CAD build for the part. Positions are in the model's coordinates, mm. Round coordinates to 2 decimals unless told otherwise and drop trailing zeros. Write each loop counter-clockwise with the first axis right and the second up, starting at its lowest first coordinate (ties: lowest second). Pieces come first, ordered by that corner, then holes. Notation, with made-up numbers: (-19, 39.25) - (39, 39.25) arc R14 cw to (39, 64.25) - close; hole circle Ø8 at (-2, -10.75). An arc over 180 degrees is marked (long way). Put each result on its own line as item: value. Start each with the question number.
Item 1: Cut at C-C (z = 2.4). Give the cut face in (x, y) (3 decimals).
Item 2: Drill centre lines: line 1 (Y direction, x = -12.15, z = 2.1) (3 decimals); line 2 (Y direction, x = -5.5, z = 0.6); line 3 (X direction, y = 32.5, z = 3.7). Where is each one in solid material? Low to high. Write a range as from..to.
Item 3: Mould opens along X. For faces 1 (the cylindrical face through (-6.076, 34.294, 2.528)), 2 (the flat face through (-4, 9.751, 2)), 3 (the cylindrical face through (-12.38, 33.26, 2.47)) say: released by +X, released by -X, zero draft, split by the parting line, or undercut.
Item 4: Cut at A-A (x = -12.15). Give the cut face in (y, z) (3 decimals), and give its area (3 significant figures).
Item 5: Cut at B-B (y = 6). Give the cut face in (x, z).
Item 6: Pin check, flat tips, straight feed: pin 1 Ø1.2 at (x, z) = (-4, 3) entering from -Y; pin 2 Ø4 at (x, y) = (-4, 12.49) entering from +Z; pin 3 Ø2 at (y, z) = (4.5, 2) entering from +X. Stop position of each tip, or through.
Item 7: Cut at D-D (x = -4). Give the cut face in (y, z), and give its area (3 significant figures).
```python
from build123d import *

# Parameters (mm, degrees)
SKIZZE1_R                       = 1.8
AUFSATZ_LINEAR_AUSTRAGEN1_DEPTH = 5
VERRUNDUNG1_R                   = 2
FASE1_SIZE                      = 0.5


with BuildPart() as part:
    # Skizze1 → Aufsatz-Linear austragen1 (new body)
    with BuildSketch(Plane.XY):
        Polygon((-0.2, 9.751346921), (-0.2, 28.627239348), (-6.022760652, 34.45), (-16.1, 34.45), (-16.1, 0.2), (-8.2, 0.2), (-8.2, 9.751346921), align=None)
        with Locations((-12.15, 31.475)):
            Circle(SKIZZE1_R, mode=Mode.SUBTRACT)
        with Locations((-4, 12.49111782)):
            Circle(SKIZZE1_R, mode=Mode.SUBTRACT)
    extrude(amount=AUFSATZ_LINEAR_AUSTRAGEN1_DEPTH)

    # Verrundung1
    verrundung1_edges = [part.edges().sort_by_distance(p)[0] for p in [
        (-8.2, 9.751346921, 2.5),
        (-8.2, 0.2, 2.5),
        (-16.1, 0.2, 2.5),
        (-16.1, 34.45, 2.5),
        (-6.022760652, 34.45, 2.5),
        (-0.2, 28.627239348, 2.5),
        (-0.2, 9.751346921, 2.5),
    ]]
    fillet(verrundung1_edges, radius=VERRUNDUNG1_R)

    # Fase1
    # the kernel refuses this chamfer: 0.5 mm, written as the material it takes off along each edge
    with BuildSketch(Plane(origin=(-12.15, 31.475, 0), x_dir=(1, 0, 0), z_dir=(0, -1, 0))) as fase1_piece_1:
        Polygon((1.8 + FASE1_SIZE, 0), (1.8, FASE1_SIZE), (1.8, 0), align=None)
    revolve(axis=Axis((-12.15, 31.475, 0), (0, 0, 1)), mode=Mode.SUBTRACT)
    with BuildSketch(Plane(origin=(-12.15, 31.475, 5), x_dir=(1, 0, 0), z_dir=(0, -1, 0))) as fase1_piece_2:
        Polygon((1.8 + FASE1_SIZE, 0), (1.8, -FASE1_SIZE), (1.8, 0), align=None)
    revolve(axis=Axis((-12.15, 31.475, 5), (0, 0, 1)), mode=Mode.SUBTRACT)
    with BuildSketch(Plane(origin=(-4, 12.49111782, 0), x_dir=(1, 0, 0), z_dir=(0, -1, 0))) as fase1_piece_3:
        Polygon((1.8 + FASE1_SIZE, 0), (1.8, FASE1_SIZE), (1.8, 0), align=None)
    revolve(axis=Axis((-4, 12.49111782, 0), (0, 0, 1)), mode=Mode.SUBTRACT)
    with BuildSketch(Plane(origin=(-4, 12.49111782, 5), x_dir=(1, 0, 0), z_dir=(0, -1, 0))) as fase1_piece_4:
        Polygon((1.8 + FASE1_SIZE, 0), (1.8, -FASE1_SIZE), (1.8, 0), align=None)
    revolve(axis=Axis((-4, 12.49111782, 5), (0, 0, 1)), mode=Mode.SUBTRACT)
    with BuildSketch(Plane(origin=(-0.2, 11.751346921, 0), x_dir=(0.027495876610586382, 0, 0.9996219169112968), z_dir=(0, 1, 0))) as fase1_piece_5:
        Polygon((FASE1_SIZE * 0.999621916911, -FASE1_SIZE * 0.0274958766106), (-FASE1_SIZE * 0.0274958766106, -FASE1_SIZE * 0.999621916911), (0, 0), align=None)
    extrude(amount=16.047465302, mode=Mode.SUBTRACT)
    with BuildSketch(Plane(origin=(-0.2, 11.751346921, 5), x_dir=(0.027495876610586403, 0, -0.9996219169112968), z_dir=(0, 1, 0))) as fase1_piece_6:
        Polygon((FASE1_SIZE * 0.999621916911, FASE1_SIZE * 0.0274958766106), (-FASE1_SIZE * 0.0274958766106, FASE1_SIZE * 0.999621916911), (0, 0), align=None)
    extrude(amount=16.047465302, mode=Mode.SUBTRACT)
    with BuildSketch(Plane(origin=(-6.2, 9.751346921, 0), x_dir=(0, 0.9996219169112968, -0.02749587661058639), z_dir=(1, 0, 0))) as fase1_piece_7:
        Polygon((FASE1_SIZE * 0.999621916911, FASE1_SIZE * 0.0274958766106), (-FASE1_SIZE * 0.0274958766106, FASE1_SIZE * 0.999621916911), (0, 0), align=None)
    extrude(amount=4, mode=Mode.SUBTRACT)
    with BuildSketch(Plane(origin=(-8.2, 2.2, 0), x_dir=(-0.9996219169112968, 0, -0.02749587661058639), z_dir=(0, 1, 0))) as fase1_piece_8:
        Polygon((FASE1_SIZE * 0.999621916911, FASE1_SIZE * 0.0274958766106), (-FASE1_SIZE * 0.0274958766106, FASE1_SIZE * 0.999621916911), (0, 0), align=None)
    extrude(amount=5.551346921, mode=Mode.SUBTRACT)
    with BuildSketch(Plane(origin=(-14.1, 0.2, 0), x_dir=(0, 0.9996219169112968, -0.027495876610586372), z_dir=(1, 0, 0))) as fase1_piece_9:
        Polygon((FASE1_SIZE * 0.999621916911, FASE1_SIZE * 0.0274958766106), (-FASE1_SIZE * 0.0274958766106, FASE1_SIZE * 0.999621916911), (0, 0), align=None)
    extrude(amount=3.9, mode=Mode.SUBTRACT)
    with BuildSketch(Plane(origin=(-16.1, 32.45, 0), x_dir=(0.9996219169112968, 0, -0.02749587661058639), z_dir=(0, -1, 0))) as fase1_piece_10:
        Polygon((FASE1_SIZE * 0.999621916911, FASE1_SIZE * 0.0274958766106), (-FASE1_SIZE * 0.0274958766106, FASE1_SIZE * 0.999621916911), (0, 0), align=None)
    extrude(amount=30.25, mode=Mode.SUBTRACT)
    with BuildSketch(Plane(origin=(-6.851187777, 34.45, 0), x_dir=(0, -0.9996219169112968, -0.027495876610586483), z_dir=(-1, 0, 0))) as fase1_piece_11:
        Polygon((FASE1_SIZE * 0.999621916911, FASE1_SIZE * 0.0274958766106), (-FASE1_SIZE * 0.0274958766106, FASE1_SIZE * 0.999621916911), (0, 0), align=None)
    extrude(amount=7.248812223, mode=Mode.SUBTRACT)
    with BuildSketch(Plane(origin=(-0.785786438, 29.213025785, 0), x_dir=(-0.7068394360706736, -0.7068394360706733, -0.027495876610586348), z_dir=(-0.7071067811865475, 0.7071067811865477, 0))) as fase1_piece_12:
        Polygon((FASE1_SIZE * 0.999621916911, FASE1_SIZE * 0.0274958766106), (-FASE1_SIZE * 0.0274958766106, FASE1_SIZE * 0.999621916911), (0, 0), align=None)
    extrude(amount=6.577772835, mode=Mode.SUBTRACT)
    with BuildSketch(Plane(origin=(-2.2, 27.798812223, 0), x_dir=(1, 0, 0), z_dir=(0, -1, 0))) as fase1_piece_13:
        Polygon((2 - FASE1_SIZE, 0), (2, FASE1_SIZE), (2, 0), align=None)
    revolve(axis=Axis((-2.2, 27.798812223, 0), (0, 0, 1)), revolution_arc=45, mode=Mode.SUBTRACT)
    with BuildSketch(Plane(origin=(-6.851187777, 32.45, 0), x_dir=(0.7071067811865487, 0.7071067811865465, 0), z_dir=(0.7071067811865465, -0.7071067811865487, 0))) as fase1_piece_14:
        Polygon((2 - FASE1_SIZE, 0), (2, FASE1_SIZE), (2, 0), align=None)
    revolve(axis=Axis((-6.851187777, 32.45, 0), (0, 0, 1)), revolution_arc=45, mode=Mode.SUBTRACT)
    with BuildSketch(Plane(origin=(-14.1, 32.45, 0), x_dir=(0, 1, 0), z_dir=(1, 0, 0))) as fase1_piece_15:
        Polygon((2 - FASE1_SIZE, 0), (2, FASE1_SIZE), (2, 0), align=None)
    revolve(axis=Axis((-14.1, 32.45, 0), (0, 0, 1)), revolution_arc=90, mode=Mode.SUBTRACT)
    with BuildSketch(Plane(origin=(-14.1, 2.2, 0), x_dir=(-1, 0, 0), z_dir=(0, 1, 0))) as fase1_piece_16:
        Polygon((2 - FASE1_SIZE, 0), (2, FASE1_SIZE), (2, 0), align=None)
    revolve(axis=Axis((-14.1, 2.2, 0), (0, 0, 1)), revolution_arc=90, mode=Mode.SUBTRACT)
    with BuildSketch(Plane(origin=(-10.2, 2.2, 0), x_dir=(0, -1, 0), z_dir=(-1, 0, 0))) as fase1_piece_17:
        Polygon((2 - FASE1_SIZE, 0), (2, FASE1_SIZE), (2, 0), align=None)
    revolve(axis=Axis((-10.2, 2.2, 0), (0, 0, 1)), revolution_arc=90, mode=Mode.SUBTRACT)
    with BuildSketch(Plane(origin=(-2.2, 11.751346921, 0), x_dir=(1, 0, 0), z_dir=(0, 1, 0))) as fase1_piece_18:
        Polygon((2 - FASE1_SIZE, 0), (2, -FASE1_SIZE), (2, 0), align=None)
    revolve(axis=Axis((-2.2, 11.751346921, 0), (0, 0, -1)), revolution_arc=90, mode=Mode.SUBTRACT)
    with BuildSketch(Plane(origin=(-6.2, 9.751346921, 5), x_dir=(0, 0.9996219169112968, 0.027495876610585647), z_dir=(1, 0, 0))) as fase1_piece_19:
        Polygon((FASE1_SIZE * 0.999621916911, -FASE1_SIZE * 0.0274958766106), (-FASE1_SIZE * 0.0274958766106, -FASE1_SIZE * 0.999621916911), (0, 0), align=None)
    extrude(amount=4, mode=Mode.SUBTRACT)
    with BuildSketch(Plane(origin=(-0.785786438, 29.213025785, 5), x_dir=(-0.7068394360706736, -0.7068394360706733, 0.027495876610585605), z_dir=(-0.7071067811865475, 0.7071067811865477, 0))) as fase1_piece_20:
        Polygon((FASE1_SIZE * 0.999621916911, -FASE1_SIZE * 0.0274958766106), (-FASE1_SIZE * 0.0274958766106, -FASE1_SIZE * 0.999621916911), (0, 0), align=None)
    extrude(amount=6.577772835, mode=Mode.SUBTRACT)
    with BuildSketch(Plane(origin=(-6.851187777, 34.45, 5), x_dir=(0, -0.9996219169112968, 0.02749587661058574), z_dir=(-1, 0, 0))) as fase1_piece_21:
        Polygon((FASE1_SIZE * 0.999621916911, -FASE1_SIZE * 0.0274958766106), (-FASE1_SIZE * 0.0274958766106, -FASE1_SIZE * 0.999621916911), (0, 0), align=None)
    extrude(amount=7.248812223, mode=Mode.SUBTRACT)
    with BuildSketch(Plane(origin=(-16.1, 32.45, 5), x_dir=(0.9996219169112968, 0, 0.027495876610585647), z_dir=(0, -1, 0))) as fase1_piece_22:
        Polygon((FASE1_SIZE * 0.999621916911, -FASE1_SIZE * 0.0274958766106), (-FASE1_SIZE * 0.0274958766106, -FASE1_SIZE * 0.999621916911), (0, 0), align=None)
    extrude(amount=30.25, mode=Mode.SUBTRACT)
    with BuildSketch(Plane(origin=(-14.1, 0.2, 5), x_dir=(0, 0.9996219169112968, 0.02749587661058563), z_dir=(1, 0, 0))) as fase1_piece_23:
        Polygon((FASE1_SIZE * 0.999621916911, -FASE1_SIZE * 0.0274958766106), (-FASE1_SIZE * 0.0274958766106, -FASE1_SIZE * 0.999621916911), (0, 0), align=None)
    extrude(amount=3.9, mode=Mode.SUBTRACT)
    with BuildSketch(Plane(origin=(-8.2, 2.2, 5), x_dir=(-0.9996219169112968, 0, 0.027495876610585647), z_dir=(0, 1, 0))) as fase1_piece_24:
        Polygon((FASE1_SIZE * 0.999621916911, -FASE1_SIZE * 0.0274958766106), (-FASE1_SIZE * 0.0274958766106, -FASE1_SIZE * 0.999621916911), (0, 0), align=None)
    extrude(amount=5.551346921, mode=Mode.SUBTRACT)
    with BuildSketch(Plane(origin=(-2.2, 27.798812223, 5), x_dir=(1, 0, 0), z_dir=(0, -1, 0))) as fase1_piece_25:
        Polygon((2, -FASE1_SIZE), (2 - FASE1_SIZE, 0), (2, 0), align=None)
    revolve(axis=Axis((-2.2, 27.798812223, 5), (0, 0, 1)), revolution_arc=45, mode=Mode.SUBTRACT)
    with BuildSketch(Plane(origin=(-6.851187777, 32.45, 5), x_dir=(0.7071067811865487, 0.7071067811865465, 0), z_dir=(0.7071067811865465, -0.7071067811865487, 0))) as fase1_piece_26:
        Polygon((2 - FASE1_SIZE, 0), (2, -FASE1_SIZE), (2, 0), align=None)
    revolve(axis=Axis((-6.851187777, 32.45, 5), (0, 0, 1)), revolution_arc=45, mode=Mode.SUBTRACT)
    with BuildSketch(Plane(origin=(-14.1, 32.45, 5), x_dir=(0, 1, 0), z_dir=(1, 0, 0))) as fase1_piece_27:
        Polygon((2 - FASE1_SIZE, 0), (2, -FASE1_SIZE), (2, 0), align=None)
    revolve(axis=Axis((-14.1, 32.45, 5), (0, 0, 1)), revolution_arc=90, mode=Mode.SUBTRACT)
    with BuildSketch(Plane(origin=(-14.1, 2.2, 5), x_dir=(-1, 0, 0), z_dir=(0, 1, 0))) as fase1_piece_28:
        Polygon((2 - FASE1_SIZE, 0), (2, -FASE1_SIZE), (2, 0), align=None)
    revolve(axis=Axis((-14.1, 2.2, 5), (0, 0, 1)), revolution_arc=90, mode=Mode.SUBTRACT)
    with BuildSketch(Plane(origin=(-10.2, 2.2, 5), x_dir=(0, -1, 0), z_dir=(-1, 0, 0))) as fase1_piece_29:
        Polygon((2 - FASE1_SIZE, 0), (2, -FASE1_SIZE), (2, 0), align=None)
    revolve(axis=Axis((-10.2, 2.2, 5), (0, 0, 1)), revolution_arc=90, mode=Mode.SUBTRACT)
    with BuildSketch(Plane(origin=(-2.2, 11.751346921, 5), x_dir=(1, 0, 0), z_dir=(0, 1, 0))) as fase1_piece_30:
        Polygon((2, FASE1_SIZE), (2 - FASE1_SIZE, 0), (2, 0), align=None)
    revolve(axis=Axis((-2.2, 11.751346921, 5), (0, 0, -1)), revolution_arc=90, mode=Mode.SUBTRACT)
    with BuildSketch(Plane(origin=(-6.2, 7.751346921, 0), x_dir=(-1, 0, 0), z_dir=(0, -1, 0))) as fase1_piece_31:
        Polygon((2 + FASE1_SIZE, 0), (2, -FASE1_SIZE), (2, 0), align=None)
    revolve(axis=Axis((-6.2, 7.751346921, 0), (0, 0, -1)), revolution_arc=90, mode=Mode.SUBTRACT)
    with BuildSketch(Plane(origin=(-6.2, 7.751346921, 5), x_dir=(-1, 0, 0), z_dir=(0, -1, 0))) as fase1_piece_32:
        Polygon((2 + FASE1_SIZE, 0), (2, FASE1_SIZE), (2, 0), align=None)
    revolve(axis=Axis((-6.2, 7.751346921, 5), (0, 0, -1)), revolution_arc=90, mode=Mode.SUBTRACT)


solid = part.part
```
Output values:
1. outline: (-16.1, 2.2) arc R2 ccw to (-14.1, 0.2) - (-10.2, 0.2) arc R2 ccw to (-8.2, 2.2) - (-8.2, 7.751) arc R2 cw to (-6.2, 9.751) - (-2.2, 9.751) arc R2 ccw to (-0.2, 11.751) - (-0.2, 27.799) arc R2 ccw to (-0.786, 29.213) - (-5.437, 33.864) arc R2 ccw to (-6.851, 34.45) - (-14.1, 34.45) arc R2 ccw to (-16.1, 32.45) - close; hole circle Ø3.6 at (-12.15, 31.475); hole circle Ø3.6 at (-4, 12.491)
2. line 1: 0.2..29.675, 33.275..34.45
2. line 2: 9.75..11.5, 13.49..33.92
2. line 3: -16.1..-13.63, -10.67..-4.07
3. face 1: released by +X
3. face 2: zero draft
3. face 3: undercut
4. outline: (0.2, 0.5) - (0.7, 0) - (29.175, 0) - (29.675, 0.5) - (29.675, 4.5) - (29.175, 5) - (0.7, 5) - (0.2, 4.5) - close; (33.275, 0.5) - (33.775, 0) - (33.95, 0) - (34.45, 0.5) - (34.45, 4.5) - (33.95, 5) - (33.775, 5) - (33.275, 4.5) - close
4. area: 152 mm2
5. outline: (-16.1, 0.5) - (-15.6, 0) - (-8.7, 0) - (-8.2, 0.5) - (-8.2, 4.5) - (-8.7, 5) - (-15.6, 5) - (-16.1, 4.5) - close
6. pin 1: y = 9.75
6. pin 2: z = 4.7
6. pin 3: x = -8.2
7. outline: (9.75, 0.5) - (10.22, 0.03) - (10.69, 0.5) - (10.69, 4.5) - (10.22, 4.97) - (9.75, 4.5) - close; (14.29, 0.5) - (14.79, 0) - (31.72, 0) - (32.43, 0.5) - (32.43, 4.5) - (31.72, 5) - (14.79, 5) - (14.29, 4.5) - close
7. area: 94.3 mm2
